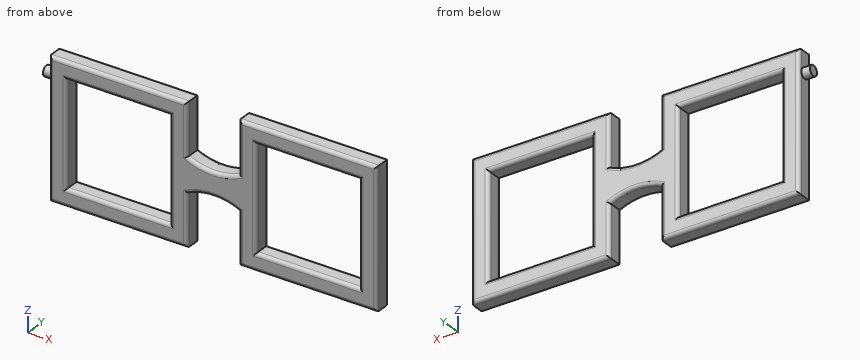
from build123d import *

# Parameters (mm, degrees)
F0_W     = 38.1
F0_H     = 38.1
F1_DEPTH = 6.35
F4_DEPTH = 6.35
F5_DEPTH = 6.351
F2_R     = 1.905
F6_DEPTH = 3.175
F7_R     = 1.26999


# Not quite as in the source:
# - a fillet or chamfer is up to 0.001 mm smaller than in the source, because OpenCascade refuses the exact size
# - a feature names something its author has since deleted; it is built from what else it names


with BuildPart() as f1:
    # F0 (on Front) → F1 (new body)
    with BuildSketch(Plane.XZ):
        Polygon((0, 12.7), (0, 31.75), (-50.8, 31.75), (-50.8, -19.05), (0, -19.05), (0, 0), (19.05, 0), (19.05, -19.05), (69.85, -19.05), (69.85, 31.75), (19.05, 31.75), (19.05, 12.7), align=None)
        with Locations((-25.4, 6.35)):
            Rectangle(F0_W, F0_H, mode=Mode.SUBTRACT)
        with Locations((44.45, 6.35)):
            Rectangle(F0_W, F0_H, mode=Mode.SUBTRACT)
    extrude(amount=F1_DEPTH)

    # F3 (on face) → F4 (join)
    with BuildSketch(Plane.XZ.offset(6.35)):
        with BuildLine():
            Line((0, 0), (19.05, 0))
            ThreePointArc((19.05, 0), (9.525, 2.0789034216), (0, 0))
        make_face()
        with BuildLine():
            Line((19.05, 12.7), (0, 12.7))
            ThreePointArc((0, 12.7), (9.525, 10.6210965784), (19.05, 12.7))
        make_face()
    extrude(amount=-F4_DEPTH)

    # F3 (on face) → F5 (cut, through all)
    with BuildSketch(Plane.XZ.offset(6.35)):
        with BuildLine():
            Line((0, 0), (19.05, 0))
            ThreePointArc((19.05, 0), (9.525, 2.0789034216), (0, 0))
        make_face()
        with BuildLine():
            Line((19.05, 12.7), (0, 12.7))
            ThreePointArc((0, 12.7), (9.525, 10.6210965784), (19.05, 12.7))
        make_face()
    extrude(amount=-F5_DEPTH, mode=Mode.SUBTRACT)

    # F2 (on face) → F6 (join, symmetric)
    with BuildSketch(Plane(origin=(-50.8, 0, 0), x_dir=(0, -1, 0), z_dir=(-1, 0, 0))):
        with Locations((3.175, 24.13)):
            Circle(F2_R)
    extrude(amount=F6_DEPTH, both=True)

    # F7 (radius 1.27 in the source; OpenCascade refuses exactly that, so slightly less here)
    f7_edges = [f1.edges().sort_by_distance(p)[0] for p in [
        (-25.4, -6.35, 31.75),
        (-50.8, -6.35, 6.35),
        (-25.4, -6.35, -19.05),
        (0, -6.35, -9.525),
        (0, -6.35, 22.225),
        (19.05, -6.35, 22.225),
        (19.05, -6.35, -9.525),
        (44.45, -6.35, -19.05),
        (69.85, -6.35, 6.35),
        (44.45, -6.35, 31.75),
        (44.45, 0, 31.75),
        (19.05, 0, 22.225),
        (0, 0, 22.225),
        (-25.4, 0, 31.75),
        (-50.8, 0, 6.35),
        (-25.4, 0, -19.05),
        (0, 0, -9.525),
        (19.05, 0, -9.525),
        (44.45, 0, -19.05),
        (69.85, 0, 6.35),
        (9.525, -6.35, 10.621097),
        (9.525, 0, 10.621097),
        (9.525, 0, 2.078903),
        (9.525, -6.35, 2.078903),
        (25.4, -6.35, 6.35),
        (25.4, 0, 6.35),
        (44.45, -6.35, -12.7),
        (44.45, 0, -12.7),
        (63.5, -6.35, 6.35),
        (63.5, 0, 6.35),
        (44.45, 0, 25.4),
        (44.45, -6.35, 25.4),
        (-25.4, -6.35, 25.4),
        (-25.4, 0, 25.4),
        (-44.45, 0, 6.35),
        (-44.45, -6.35, 6.35),
        (-25.4, 0, -12.7),
        (-25.4, -6.35, -12.7),
        (-6.35, 0, 6.35),
        (-6.35, -6.35, 6.35),
    ]]
    fillet(f7_edges, radius=F7_R)


solid = f1.part
Here's how the part is built. I have some questions about the finished solid (model axes, mm). Round coordinates to 2 decimals unless told otherwise and drop trailing zeros. Loops run counter-clockwise (first coordinate to the right, second up) from the corner with the lowest first, then second, coordinate; pieces in that order, holes last. Notation, with made-up numbers: (18.5, 8) -> (69.5, 8) arc R26 cw to (69.5, 41) -> close; hole circle Ø8 at (23.5, 35). An arc over 180 degrees is marked (long way). Write each question's results on one line, items separated by ' | '.
(1) If we section it at B-B, the plane y = -2.5: List the corners of the cut face in (x, z) for me (3 decimals).
Worked answers:
outline: (-53.975, 22.349) -> (-50.8, 22.349) -> (-50.8, -19.05) -> (0, -19.05) -> (0, 0) arc R22.86 cw to (19.05, 0) -> (19.05, -19.05) -> (69.85, -19.05) -> (69.85, 31.75) -> (19.05, 31.75) -> (19.05, 12.7) arc R22.86 cw to (0, 12.7) -> (0, 31.75) -> (-50.8, 31.75) -> (-50.8, 25.911) -> (-53.975, 25.911) -> close; hole (-44.45, -12.7) -> (-6.35, -12.7) -> (-6.35, 25.4) -> (-44.45, 25.4) -> close; hole (25.4, -12.7) -> (63.5, -12.7) -> (63.5, 25.4) -> (25.4, 25.4) -> close
(2) For P1, Ø5, axis at x = 1.5, z = -9, coming from the +Y side; P2, Ø1.9, axis at y = -4, z = 16, coming from the -X side, each with a flat end and sliding along its axis, tell me the tip position at first contact or that it passes through.
Worked answers:
P1: y = -0.03 | P2: x = -50.8
(3) If I drill on L1, parallel to X at y = -3.75, z = 7.5; L2, parallel to X at y = -3.5, z = 0; L3, parallel to Z at x = 41.5, y = -1.5, over which ranges is the centre line in solid material (lowest first)?
Worked answers:
L1: -50.8 to -44.45, -6.35 to 25.4, 63.5 to 69.85 | L2: -50.8 to -44.45, -6.35 to 0, 19.05 to 25.4, 63.5 to 69.85 | L3: -19.05 to -12.7, 25.4 to 31.75
(4) If we section it at A-A, the plane z = -4: Give the number of separate pieces and of enclosed holes in the cut face, then the cut area to 3 significant figures.
Worked answers:
separate pieces: 4 | enclosed holes: 0 | area: 156 mm2
